Design review of the part built by this model. Coordinates are the model's own, in mm. Give positions to 0.01 mm unless a question says otherwise; leave off trailing zeros. Write each loop counter-clockwise with the first axis right and the second up, starting at its lowest first coordinate (ties: lowest second). Pieces come first, ordered by that corner, then holes. Notation, with made-up numbers: M -18.5,51 L -3.5,51 A14 cw -3.5,72 Z; hole C 40.5,72.5 d8. An arc over 180 degrees is marked long. Answer in a Markdown table with one row per item.
```python
from build123d import *

# Parameters (mm, degrees)
SKETCH_R   = 3
SKETCH_R_2 = 4.5
PAD_DEPTH  = 4


with BuildPart() as part:
    # Sketch → Pad (new body)
    with BuildSketch(Plane.XY):
        with BuildLine():
            Line((0, 119.313708), (0, -119.313708))
            ThreePointArc((0, -119.313708), (1.234633, -121.161468), (3.414214, -120.727922))
            Line((3.414214, -120.727922), (19.414214, -104.727922))
            ThreePointArc((19.414214, -104.727922), (19.847759, -104.079075), (20, -103.313708))
            Line((20, -50), (20, -103.313708))
            ThreePointArc((20.585786, -48.585786), (20.152241, -49.234633), (20, -50))
            Line((20.585786, -48.585786), (58.585786, -10.585786))
            ThreePointArc((60, -10), (59.234633, -10.152241), (58.585786, -10.585786))
            Line((60, -10), (113.313708, -10))
            ThreePointArc((113.313708, -10), (114.079075, -9.847759), (114.727922, -9.414214))
            Line((114.727922, -9.414214), (122.727922, -1.414214))
            ThreePointArc((122.727922, -1.414214), (123.313708, 0), (122.727922, 1.414214))
            Line((114.727922, 9.414214), (122.727922, 1.414214))
            ThreePointArc((114.727922, 9.414214), (114.079075, 9.847759), (113.313708, 10))
            Line((113.313708, 10), (60, 10))
            ThreePointArc((58.585786, 10.585786), (59.234633, 10.152241), (60, 10))
            Line((58.585786, 10.585786), (20.585786, 48.585786))
            ThreePointArc((20, 50), (20.152241, 49.234633), (20.585786, 48.585786))
            Line((20, 50), (20, 103.313708))
            ThreePointArc((20, 103.313708), (19.847759, 104.079075), (19.414214, 104.727922))
            Line((3.414214, 120.727922), (19.414214, 104.727922))
            ThreePointArc((3.414214, 120.727922), (1.234633, 121.161468), (0, 119.313708))
        make_face()
        with Locations((10, -100)):
            Circle(SKETCH_R, mode=Mode.SUBTRACT)
        with Locations((10, 100)):
            Circle(SKETCH_R, mode=Mode.SUBTRACT)
        with Locations((110, 0)):
            Circle(SKETCH_R, mode=Mode.SUBTRACT)
        with Locations((30, 0)):
            Circle(SKETCH_R, mode=Mode.SUBTRACT)
        with Locations((30, 28)):
            Circle(SKETCH_R_2, mode=Mode.SUBTRACT)
    extrude(amount=PAD_DEPTH)


solid = part.part
```
1) Add section B-B (y = 28). Write out the cut boundary in (x, z).
Geometry says:
| item | result |
|---|---|
| outline | M 0,0 L 25.5,0 L 25.5,4 L 0,4 Z; M 34.5,0 L 41.17,0 L 41.17,4 L 34.5,4 Z |
2) Insertion check: P1, Ø3.5, axis at x = 30, y = 0, coming from the +Z side; P2, Ø1.2, axis at x = 82.5, z = 2.5, coming from the -Y side; P3, Ø1.2, axis at y = -78.5, z = 1, coming from the +X side. Each pin has a flat end and moves straight along its axis. Give the tip position at first contact, or say it passes through.
Geometry says:
| item | result |
|---|---|
| P1 | through |
| P2 | y = -10 |
| P3 | x = 20 |
3) Add section A-A (z = 2.3). Write out the cut boundary in (x, y).
Geometry says:
| item | result |
|---|---|
| outline | M 0,-119.31 A2 ccw 3.41,-120.73 L 19.41,-104.73 A2 ccw 20,-103.31 L 20,-50 A2 cw 20.59,-48.59 L 58.59,-10.59 A2 cw 60,-10 L 113.31,-10 A2 ccw 114.73,-9.41 L 122.73,-1.41 A2 ccw 122.73,1.41 L 114.73,9.41 A2 ccw 113.31,10 L 60,10 A2 cw 58.59,10.59 L 20.59,48.59 A2 cw 20,50 L 20,103.31 A2 ccw 19.41,104.73 L 3.41,120.73 A2 ccw 0,119.31 Z; hole C 10,-100 d6; hole C 10,100 d6; hole C 30,28 d9; hole C 30,0 d6; hole C 110,0 d6 |
4) Add section C-C (x = 30). Write out the cut boundary in (y, z), and give its area (3 significant figures).
Geometry says:
| item | result |
|---|---|
| outline | M -39.17,0 L -3,0 L -3,4 L -39.17,4 Z; M 3,0 L 23.5,0 L 23.5,4 L 3,4 Z; M 32.5,0 L 39.17,0 L 39.17,4 L 32.5,4 Z |
| area | 253 mm^2 |
5) Add section D-D (y = -79.5). Write out the cut boundary in (x, z), and give its area (3 significant figures).
Geometry says:
| item | result |
|---|---|
| outline | M 0,0 L 20,0 L 20,4 L 0,4 Z |
| area | 80.0 mm^2 |
6) The part is to be moulded in two halves that separate along X. For faces 1 (the face through (32.08, 24.01, 1.97)), 2 (the face through (118.67, 5.47, 1.97)), 3 (the face through (34, 1, 4)), say which applies: released by +X, released by -X, zero draft, split by the parting line, or undercut.
Geometry says:
| item | result |
|---|---|
| face 1 | undercut |
| face 2 | released by +X |
| face 3 | zero draft |
7) To check wall thickness, follow probe 1 along Y at (x, z) = (10, 1.75); probe 2 along Y at (x, z) = (29.5, 1.4); probe 3 along Y at (x, z) = (71, 0.4). State the ranges of each line that lie inside material, in increasing order. Write a range as [from, to].
Geometry says:
| item | result |
|---|---|
| probe 1 | [-114.14, -103], [-97, 97], [103, 114.14] |
| probe 2 | [-39.67, -2.96], [2.96, 23.53], [32.47, 39.67] |
| probe 3 | [-10, 10] |
